Part model, mm, in its own coordinate system. Face numbers are marked on the shaded views. A direction names the side the tool comes from. Coordinates: 2 decimals unless noted, no trailing zeros. Write each loop counter-clockwise with the first axis right and the second up, starting at its lowest first coordinate (ties: lowest second). Pieces come first, ordered by that corner, then holes. Notation, with made-up numbers: (53.25, 31.25) -> (72.25, 31.25) arc R35 ccw to (72.25, 65.25) -> close; hole circle Ø3 at (-27.5, 75.25). An arc over 180 degrees is marked (long way). Write item = value, one per line. Start each with the question number.
Q1. Pull direction Z, two halves, no side cores. Call the marked faces 1, 2 and 3: released by +Z, released by -Z, zero draft, split by the parting line, or undercut.
Q2. Band-saw the part on D-D, the plane y = 65.5. List the corners of the cut face in (x, z).
Q3. Pin check, flat tips, straight feed: P1, Ø6.5, axis at y = 7.5, z = 7.5, coming from the +X side; P2, Ø10, axis at x = -3.5, z = 48, coming from the +Y side; P3, Ø1.5, axis at y = 56, z = 85, coming from the +X side. Stop position of each tip, or through.
Q4. Tool access for the marked faces 4 and 5: list every direction of +Z, -Z, +X, -X, +Y, -Y with a clear straight run to the whole face (end or side of a thin tool).
Q5. Band-saw the part on C-C, the plane x = 32. List the corners of the cut face in (y, z), plus the area to 3 significant figures.
Q6. Band-saw the part on A-A, the plane z = 59.5. List the corners of the cut face in (x, y), plus the area to 3 significant figures.
Q7. Band-saw the part on B-B, the plane y = 7.5. Give the number of separate pieces and of enclosed holes in the cut face, plus the area to 4 significant figures.
Q8. Probe line 1 (Z direction, x = -17.4, y = 52.5); line 2 (Y direction, x = -17.2, z = -7.5); line 3 (Y direction, x = 7.5, z = -18.1). List the from-to ranges inside material, lowest first.
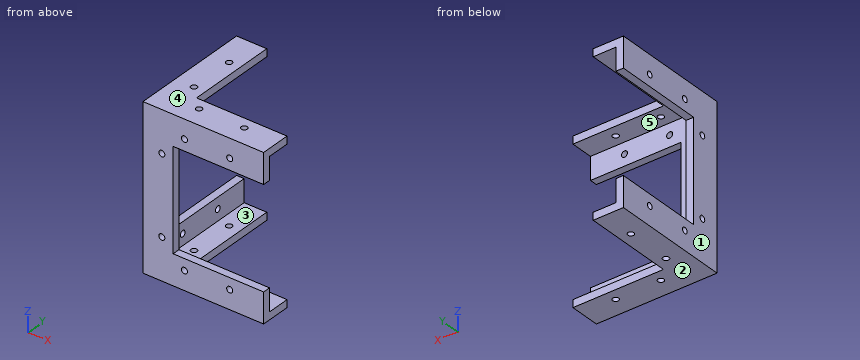
from build123d import *

# Parameters (mm, degrees)
BOSS_EXTRUDE1_DEPTH             = 5
BOSS_EXTRUDE2_DEPTH             = 5
BOSS_EXTRUDE3_DEPTH             = 5
HIEGHT_EXTENSION_DEPTH          = 27
BOSS_EXTRUDE6_DEPTH             = 5
SKETCH7_W                       = 20
SKETCH7_H                       = 80
BOSS_EXTRUDE7_DEPTH             = 5
SKETCH8_W                       = 80
SKETCH8_H                       = 20
BOSS_EXTRUDE8_DEPTH             = 5
F_4_0MM_DOWEL_HOLE1_D           = 4
F_4_0MM_DOWEL_HOLE1_ON_FACE_2_D = 4
F_4_0MM_DOWEL_HOLE1_ON_FACE_3_D = 4
F_4_0MM_DOWEL_HOLE1_ON_FACE_4_D = 4


with BuildPart() as part:
    # Sketch1 → Boss-Extrude1 (new body)
    with BuildSketch(Plane(origin=(0, 0, 0), x_dir=(1, 0, 0), z_dir=(0, 1, 0))):
        Polygon((-20, 20), (-20, -60), (0, -60), (0, 0), (60, 0), (60, 20), align=None)
    extrude(amount=-BOSS_EXTRUDE1_DEPTH)

    # Sketch2 → Boss-Extrude2 (add)
    with BuildSketch(Plane.ZY.offset(20)):
        Polygon((-20, -5), (60, -5), (60, 15), (0, 15), (0, 75), (-20, 75), align=None)
    extrude(amount=-BOSS_EXTRUDE2_DEPTH)

    # Sketch3 → Boss-Extrude3 (add)
    with BuildSketch(Plane(origin=(0, 0, -20), x_dir=(-1, 0, 0), z_dir=(0, 0, -1))):
        Polygon((-60, -5), (20, -5), (20, 75), (0, 75), (0, 15), (-60, 15), align=None)
    extrude(amount=-BOSS_EXTRUDE3_DEPTH)

    # Sketch5 → hieght extension (add)
    with BuildSketch(Plane.XY.offset(60)):
        Polygon((0, 0), (-15, 0), (-15, 15), (-20, 15), (-20, -5), (0, -5), align=None)
    extrude(amount=HIEGHT_EXTENSION_DEPTH)

    # Sketch6 → Boss-Extrude6 (add)
    with BuildSketch(Plane.XY.offset(87)):
        Polygon((-20, 75), (-20, -5), (60, -5), (60, 15), (0, 15), (0, 75), align=None)
    extrude(amount=-BOSS_EXTRUDE6_DEPTH)

    # Sketch7 → Boss-Extrude7 (add)
    with BuildSketch(Plane.ZY.offset(20)):
        with Locations((77, 35)):
            Rectangle(SKETCH7_W, SKETCH7_H)
    extrude(amount=-BOSS_EXTRUDE7_DEPTH)

    # Sketch8 → Boss-Extrude8 (add)
    with BuildSketch(Plane.XZ.offset(5)):
        with Locations((20, 77)):
            Rectangle(SKETCH8_W, SKETCH8_H)
    extrude(amount=-BOSS_EXTRUDE8_DEPTH)

    # Ø4.0mm Dowel Hole1 (through all)
    with Locations(Plane(origin=(-15, 52.5, 74.5), x_dir=(0, 0, 1), z_dir=(1, 0, 0))):
        with Locations((0, 0), (0, 30), (-67, 45), (-15, 45), (-82, 30), (-82, 0)):
            Hole(F_4_0MM_DOWEL_HOLE1_D / 2)

    # Ø4.0mm Dowel Hole1 on face 2 (through all)
    with Locations(Plane(origin=(7.5, 0, 74.5), x_dir=(0, 0, 1), z_dir=(0, 1, 0))):
        with Locations((0, 0), (0, 30), (-67, -15), (-15, -15), (-82, 0), (-82, 30)):
            Hole(F_4_0MM_DOWEL_HOLE1_ON_FACE_2_D / 2)

    # Ø4.0mm Dowel Hole1 on face 3 (through all)
    with Locations(Plane(origin=(-7.5, 52.5, 82), x_dir=(-1, 0, 0), z_dir=(0, 0, -1))):
        with Locations((0, 0), (0, -30), (-15, -45), (-45, -45)):
            Hole(F_4_0MM_DOWEL_HOLE1_ON_FACE_3_D / 2)

    # Ø4.0mm Dowel Hole1 on face 4 (through all)
    with Locations(Plane(origin=(37.5, 7.5, -15), x_dir=(1, 0, 0), z_dir=(0, 0, 1))):
        with Locations((0, 0), (-30, 0), (-45, 15), (-45, 45)):
            Hole(F_4_0MM_DOWEL_HOLE1_ON_FACE_4_D / 2)


solid = part.part
Ans:
q1.face_1 = zero draft
q1.face_2 = released by -Z
q1.face_3 = undercut
q2.outline = (-20, -20) -> (0, -20) -> (0, -15) -> (-15, -15) -> (-15, 0) -> (-20, 0) -> close; (-20, 67) -> (-15, 67) -> (-15, 82) -> (0, 82) -> (0, 87) -> (-20, 87) -> close
q3.P1 = -15
q3.P2 = 0
q3.P3 = 0
q4.face_4 = +Z, +X, -X, +Y, -Y
q4.face_5 = +X, +Y
q5.outline = (-5, -20) -> (15, -20) -> (15, -15) -> (0, -15) -> (0, 0) -> (-5, 0) -> close; (-5, 67) -> (0, 67) -> (0, 82) -> (15, 82) -> (15, 87) -> (-5, 87) -> close
q5.area = 350 mm2
q6.outline = (-20, -5) -> (-9.5, -5) -> (-9.5, 0) -> (-15, 0) -> (-15, 5.5) -> (-20, 5.5) -> close; (-20, 9.5) -> (-15, 9.5) -> (-15, 15) -> (-20, 15) -> close; (-5.5, -5) -> (0, -5) -> (0, 0) -> (-5.5, 0) -> close
q6.area = 135 mm2
q7.separate_pieces = 7
q7.enclosed_holes = 0
q7.area = 1,165 mm2
q8.line_1 = -20 to -9.5, -5.5 to 0, 67 to 72.5, 76.5 to 87
q8.line_2 = -5 to 20.5, 24.5 to 50.5, 54.5 to 75
q8.line_3 = -5 to 5.5, 9.5 to 15
